Answer from the drawing. Dimensions are ordinates in mm from the lowest x, y and z of the part. Coordinates: 2 decimals unless noted, no trailing zeros. Order: outer loops, then holes, each group sorted by start corner. A loop starts at its lowest first (then second) coordinate and runs counter-clockwise, first axis right, second up. Notation, with made-up numbers: (43.25, 43.5) - (87.25, 43.5) arc R32 ccw to (87.25, 78.5) - close; hole circle Ø1 at (-5.5, -35.75). An arc over 180 degrees is marked (long way). Use CSV: the item, a comma, the result in double quotes. Start each with the question number.
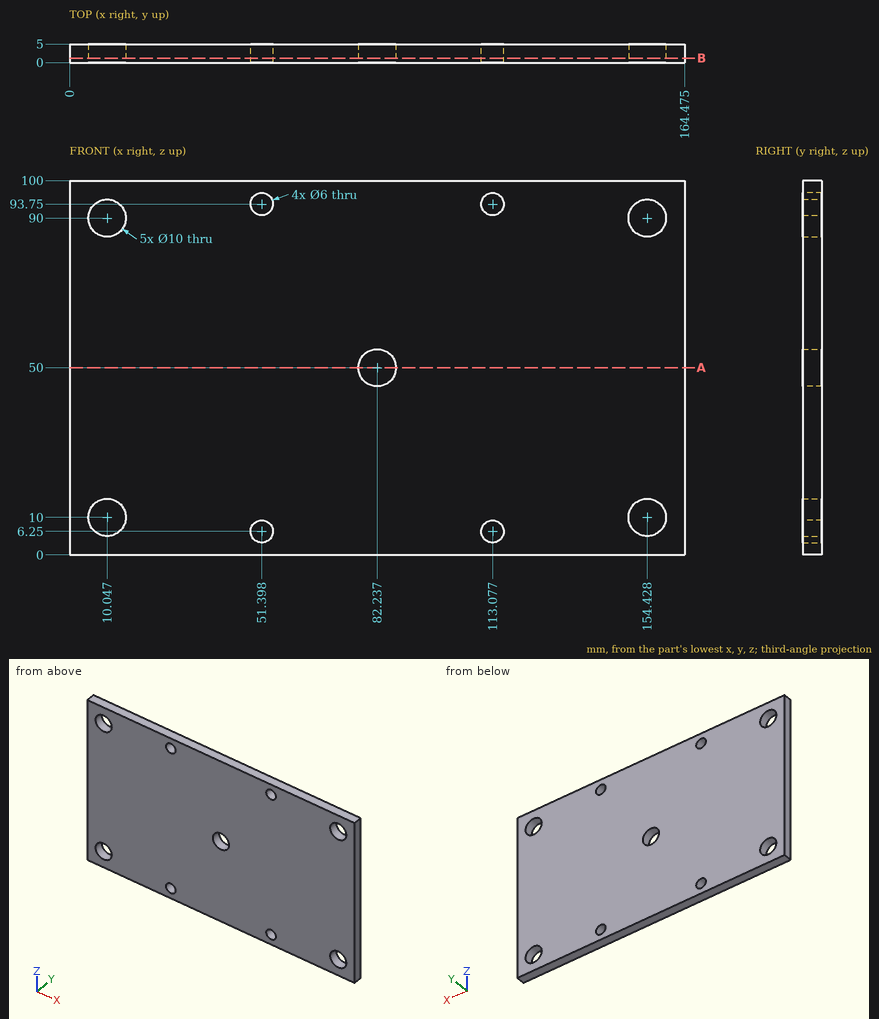
1) Straight lines are drawn through the part: line 1 (X direction, y = 1.5, z = 10) (1 decimal); line 2 (Z direction, x = 9.5, y = 2.8); line 3 (X direction, y = 3.75, z = 50) (1 decimal). For each, find the intervals that lie inside material, in ascending order. Write a range as [from, to].
2) The part is cut by section B-B on y = 1.2. State how many separate pieces and enclosed holes the cut face has, plus the area to 3 significant figures.
3) The part is cut by section A-A on z = 50. Determine the outline of the cut face in (x, y) (1 decimal).
Answer key:
1,line 1,"[0, 5], [15, 149.4], [159.4, 164.5]"
1,line 2,"[0, 5.03], [14.97, 85.03], [94.97, 100]"
1,line 3,"[0, 77.2], [87.2, 164.5]"
2,separate pieces,"1"
2,enclosed holes,"9"
2,area,"15,900 mm^2"
3,outline,"(0, 0) - (77.2, 0) - (77.2, 5) - (0, 5) - close; (87.2, 0) - (164.5, 0) - (164.5, 5) - (87.2, 5) - close"
